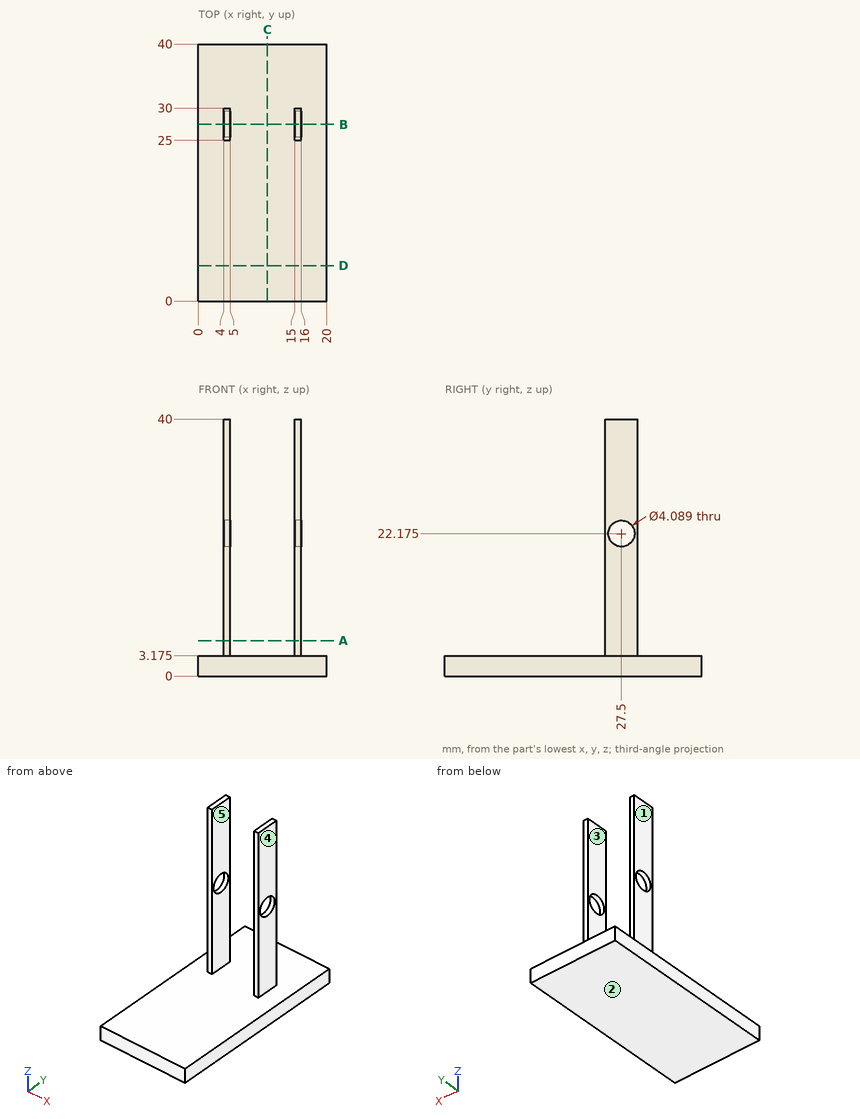
Check sheet for the drawn part. Datum: minimum x, y, z corner. Units: mm. A direction names the side the tool comes from. Round coordinates to 2 decimals unless told otherwise and drop trailing zeros. Loops run counter-clockwise (first coordinate to the right, second up) from the corner with the lowest first, then second, coordinate; pieces in that order, holes last. Notation, with made-up numbers: M 79,-0.5 L 136,-0.5 A20 ccw 136,14.5 Z; hole C 3,60.25 d5. An arc over 180 degrees is marked long. Write each question's results on one line, items separated by ' | '.
1) Section check C-C on x = 10.75. Record the boundary of the cut face in (y, z) (1 decimal).
Checks:
outline: M 0,0 L 40,0 L 40,3.2 L 0,3.2 Z
2) Access from +Z, -Z, +X, -X, +Y, -Y to the whole of each face (thin tool, end or side, straight path). Record for the marked faces 4 and 5.
Checks:
face 4: +Z, +X, +Y, -Y | face 5: +Z, +Y, -Y
3) Section check B-B on y = 27.5. Record the boundary of the cut face in (x, z) (1 decimal).
Checks:
outline: M 0,0 L 20,0 L 20,3.2 L 16,3.2 L 16,20.1 L 15,20.1 L 15,3.2 L 5,3.2 L 5,20.1 L 4,20.1 L 4,3.2 L 0,3.2 Z; M 4,24.2 L 5,24.2 L 5,40 L 4,40 Z; M 15,24.2 L 16,24.2 L 16,40 L 15,40 Z
4) Section check A-A on z = 5.5. Record the boundary of the cut face in (x, y), then the cut area to 3 significant figures.
Checks:
outline: M 4,25 L 5,25 L 5,30 L 4,30 Z; M 15,25 L 16,25 L 16,30 L 15,30 Z | area: 10.0 mm2
5) Scan lines: L1, parallel to Z at x = 15.8, y = 27.5; L2, parallel to Z at x = 12.75, y = 24.5 (1 decimal). Record each from-to range of solid material in increasing order. Write a range as from..to.
Checks:
L1: z = 0..20.13, 24.22..40 | L2: z = 0..3.2
6) Section check D-D on y = 5.5. Record the boundary of the cut face in (x, z) (1 decimal), then the cut area to 3 significant figures.
Checks:
outline: M 0,0 L 20,0 L 20,3.2 L 0,3.2 Z | area: 63.5 mm2
7) Gauge pin test, flat ends, axial feed: P1, Ø3.5, axis at y = 27.5, z = 22.175, coming from the +X side; P2, Ø10, axis at x = 7.5, z = 22.5, coming from the +Y side; P3, Ø1.5, axis at y = 27.5, z = 20.5, coming from the -X side; P4, Ø5.5, axis at y = 27, z = 28.5, coming from the +X side. Record the tip position at first contact, or that the pin passes through.
Checks:
P1: passes through | P2: stops at y = 30 | P3: stops at x = 4 | P4: stops at x = 16
8) Mould release check, pull along X, two halves, no side actions. Record for the marked faces 1, 2 and 3: released by +X, released by -X, zero draft, split by the parting line, or undercut.
Checks:
face 1: released by -X | face 2: zero draft | face 3: undercut
